Geometry: final body of the model. Coordinates: model frame, mm. Face numbers are marked on the shaded views. A direction names the side the tool comes from. Coordinates: 2 decimals unless noted, no trailing zeros. Write each loop counter-clockwise with the first axis right and the second up, starting at its lowest first coordinate (ties: lowest second). Pieces come first, ordered by that corner, then holes.
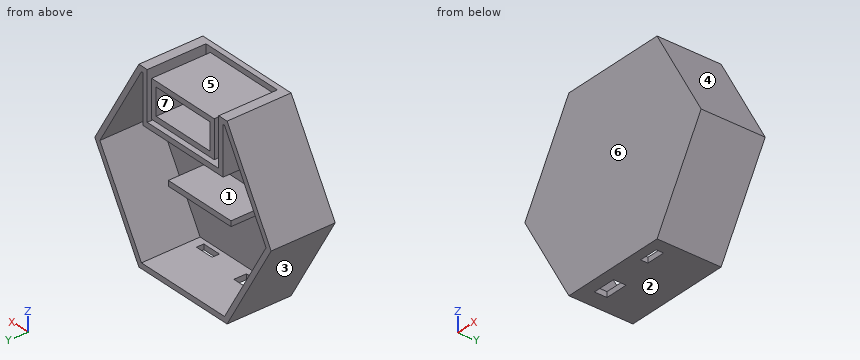
from build123d import *

# Parameters (mm, degrees)
BOSS_EXTRUDE1_DEPTH = 2.54
SKETCH3_W           = 36.089649417
SKETCH3_H           = 17.78
SKETCH3_W_2         = 31.009649417
SKETCH3_H_2         = 12.7
BOSS_EXTRUDE2_DEPTH = 30.48
SKETCH5_W           = 36.077770682
SKETCH5_H           = 2.54
BOSS_EXTRUDE3_DEPTH = 20
SKETCH7_W           = 9
SKETCH7_H           = 3.5
SKETCH7_W_2         = 11
SKETCH7_H_2         = 6
CUT_EXTRUDE1_DEPTH  = 3.54


with BuildPart() as part:
    # Sketch2 → Boss-Extrude1 (new body)
    with BuildSketch(Plane(origin=(0, 0, 0), x_dir=(1, 0, 0), z_dir=(0, 1, 0))):
        Polygon((76.2, 0), (101.6, 43.994090512), (76.2, 87.988181024), (25.4, 87.988181024), (0, 43.994090512), (25.4, 0), align=None)
    extrude(amount=BOSS_EXTRUDE1_DEPTH)

    # Sketch3 → Boss-Extrude2 (add)
    with BuildSketch(Plane(origin=(0, 0, 0), x_dir=(1, 0, 0), z_dir=(0, 1, 0))):
        with Locations((50.805939368, 11.43)):
            Rectangle(SKETCH3_W, SKETCH3_H)
        with Locations((50.805939368, 11.43)):
            Rectangle(SKETCH3_W_2, SKETCH3_H_2, mode=Mode.SUBTRACT)
        Polygon((30.221114659, 22.86), (30.221114659, 0), (25.4, 0), (0, 43.994090512), (25.4, 87.988181024), (76.2, 87.988181024), (101.6, 43.994090512), (76.2, 0), (71.390764076, 0), (71.390764076, 22.86), align=None)
        Polygon((73.930764076, 2.54), (74.733530316, 2.54), (98.667060633, 43.994090512), (74.733530316, 85.448181024), (26.866469684, 85.448181024), (2.932939367, 43.994090512), (26.866469684, 2.54), (27.681114659, 2.54), (27.681114659, 25.4), (73.930764076, 25.4), align=None, mode=Mode.SUBTRACT)
    extrude(amount=BOSS_EXTRUDE2_DEPTH)

    # Sketch5 → Boss-Extrude3 (add)
    with BuildSketch(Plane(origin=(0, 2.54, 0), x_dir=(1, 0, 0), z_dir=(0, 1, 0))):
        with Locations((50.8, 51.27)):
            Rectangle(SKETCH5_W, SKETCH5_H)
    extrude(amount=BOSS_EXTRUDE3_DEPTH)

    # Sketch7 → Cut-Extrude1 (cut, through all)
    with BuildSketch(Plane.XY.offset(-85.448181024)):
        with Locations((65.7, 6.29)):
            Rectangle(SKETCH7_W, SKETCH7_H)
        with Locations((38.9, 8.54)):
            Rectangle(SKETCH7_W_2, SKETCH7_H_2)
    extrude(amount=-CUT_EXTRUDE1_DEPTH, mode=Mode.SUBTRACT)


solid = part.part
Item 1: Section A-A, the plane y = 26. Output: boundary loops of the cut face in (x, z), plus the area to 3 significant figures.
Derived:
outline: (0, -43.99) - (25.4, -87.99) - (76.2, -87.99) - (101.6, -43.99) - (76.2, 0) - (71.39, 0) - (71.39, -22.86) - (30.22, -22.86) - (30.22, 0) - (25.4, 0) - close; (32.76, -20.32) - (68.85, -20.32) - (68.85, -2.54) - (32.76, -2.54) - close; hole (2.93, -43.99) - (26.87, -85.45) - (74.73, -85.45) - (98.67, -43.99) - (74.73, -2.54) - (73.93, -2.54) - (73.93, -25.4) - (27.68, -25.4) - (27.68, -2.54) - (26.87, -2.54) - close; hole (35.3, -17.78) - (66.31, -17.78) - (66.31, -5.08) - (35.3, -5.08) - close
area: 1,120 mm2
Item 2: Pin query (flat end, axial travel): pin 1 (3 mm diameter, centred on y = 8.5, z = -86.5, fed in from -X); pin 2 (4 mm diameter, centred on y = 21.5, z = -14.5, fed in from +X); pin 3 (11.5 mm diameter, centred on x = 56.5, z = -9, fed in from +Y); pin 4 (0.8 mm diameter, centred on y = 5.5, z = -86.5, fed in from -X). Return the tip coordinate at first contact, or that it passes through.
Derived:
pin 1: stops at x = 23.67
pin 2: stops at x = 85.73
pin 3: stops at y = 30.48
pin 4: stops at x = 24.31
Item 3: Material intervals for probe 1 along Z at (x, y) = (40, 21.5); probe 2 along Z at (x, y) = (63.5, 5); probe 3 along Z at (x, y) = (70, 16.5), sorted ascending.
Derived:
probe 1: z = -87.99 to -85.45, -52.54 to -50, -25.4 to -22.86, -20.32 to -17.78, -5.08 to -2.54
probe 2: z = -52.54 to -50, -25.4 to -22.86, -20.32 to -17.78, -5.08 to -2.54
probe 3: z = -87.99 to -85.45, -25.4 to -22.86
Item 4: Pull-direction query (X, two-part tool) for the marked faces 1, 2, 3 and 4; classes: released by +X, released by -X, zero draft, split by the parting line, or undercut.
Derived:
face 1: undercut
face 2: zero draft
face 3: released by -X
face 4: released by +X
Item 5: Section C-C, the plane x = 64. Output: boundary loops of the cut face in (y, z), plus the area to 3 significant figures.
Derived:
outline: (0, -87.99) - (4.54, -87.99) - (4.54, -85.45) - (2.54, -85.45) - (2.54, -52.54) - (22.54, -52.54) - (22.54, -50) - (2.54, -50) - (2.54, -25.4) - (30.48, -25.4) - (30.48, -22.86) - (2.54, -22.86) - (2.54, -20.32) - (30.48, -20.32) - (30.48, -17.78) - (2.54, -17.78) - (2.54, -5.08) - (30.48, -5.08) - (30.48, -2.54) - (2.54, -2.54) - (2.54, 0) - (0, 0) - close; (8.04, -87.99) - (30.48, -87.99) - (30.48, -85.45) - (8.04, -85.45) - close
area: 549 mm2
Item 6: Set-up query: the marked faces 5, 6 and 7. Return all of +Z, -Z, +X, -X, +Y, -Y with unobstructed straight access to the full face (end or side cutting, diameter ignored); none if empty.
Derived:
face 5: +Z, +Y
face 6: +Z, -Z, +X, -X, -Y
face 7: +Y
Item 7: Section B-B, the plane y = 19. State how many separate pieces and enclosed holes the cut face has, plus the area to 3 significant figures.
Derived:
separate pieces: 3
enclosed holes: 2
area: 1,210 mm2
